For this review, take the finished solid that the model builds, in its own axes (mm). A direction names the side the tool comes from. Coordinates: 2 decimals unless noted, no trailing zeros. Write each loop counter-clockwise with the first axis right and the second up, starting at its lowest first coordinate (ties: lowest second). Pieces come first, ordered by that corner, then holes.
1) To check wall thickness, follow line 1 along Y through (x, z) = (69, 13); line 2 along Y through (x, z) = (42.5, 9); line 3 along Y through (x, z) = (98, 10). State the ranges of each line that lie inside material, in increasing order.
2) We need section A-A on x = 34.5. Write out the cut boundary in (y, z).
3) We need section C-C on y = -19. Write out the cut boundary in (x, z).
4) Mouldability with a two-part tool opening along Y and no side actions: class faces 4 (the face through (61.229, -27, -9)), 5 (the face through (19, -25.416, -7)), 6 (the face through (65, -20, -13.721)), 7 (the face through (65, 58.95, 14)) as pulls with the +Y half, pulls with the -Y half, needs draft (parallel to the pull), parting line crosses it, or undercut.
5) Insertion check: P1, Ø4, axis at x = 103, z = 23.5, coming from the +Y side; P2, Ø11.5, axis at x = 33.5, y = -24.5, coming from the +Z side; P3, Ø4, axis at x = 95, y = 44.5, coming from the +Z side. Each pin has a flat end and moves straight along its axis. Give the tip position at first contact, or say it passes through.
6) We need section B-B on z = 4.5. Write out the cut boundary in (x, y), then the cut area to 3 significant figures.
7) For faces 1 (the face through (113, -25.416, -7)), 2 (the face through (34, -22.914, -1)), 3 (the face through (59.601, -27, -9)), list the 3-axis set-ups (+Z, -Z, +X, -X, +Y, -Y) from which the entire face can be reached by the end or side of a thin tool; tool diameter is ignored.
8) We need section D-D on z = 30. Write out the cut boundary in (x, y).
from build123d import *

# Parameters (mm, degrees)
F1_DEPTH  = 132.11009
F2_W      = 132.11009
F2_H      = 1.6692737117
F3_DEPTH  = 14.2200058326
F4_W      = 5.6164497176
F4_H      = 5.6164497176
F5_DEPTH  = 24.97072611
F4_W_2    = 1.6288390616
F4_H_2    = 3.1137447804
F6_DEPTH  = 10
F7_W      = 3.1137447804
F7_H      = 1.2358725164
F8_DEPTH  = 57.6303704236
F9_W      = 3.1137447804
F9_H      = 1.2358725164
F10_DEPTH = 26.006960353


with BuildPart() as f1:
    # F0 (on Right) → F1 (new body)
    with BuildSketch(Plane.YZ):
        Polygon((-41.4899997413, 44.3699993193), (-28.5300053656, 44.3699993193), (58.9500032365, 44.3699993193), (71.9099976122, 44.3699993193), (15.2099989355, 73.1699988246), align=None)
        Polygon((-14.309999533, 11.2499995157), (-14.309999533, -15.3900003061), (58.9500032365, -15.3900003061), (58.9500032365, 44.3699993193), (-28.5300053656, 44.3699993193), (-28.5300053656, 11.2499995157), align=None)
    extrude(amount=F1_DEPTH)

    # F2 (on face) → F3 (join, through all)
    with BuildSketch(Plane.XZ.offset(14.309999533)):
        with Locations((66.055045, -14.5553634502)):
            Rectangle(F2_W, F2_H)
    extrude(amount=F3_DEPTH)

    # F4 (on face) → F5 (join, through all)
    with BuildSketch(Plane.XY.offset(-13.7207265943)):
        with Locations((2.8082248588, -25.7217805068)):
            Rectangle(F4_W, F4_H)
        with Locations((34.4316349294, -25.7217805068)):
            Rectangle(F4_W, F4_H)
        with Locations((66.055045, -25.7217805068)):
            Rectangle(F4_W, F4_H)
        with Locations((97.6784550706, -25.7217805068)):
            Rectangle(F4_W, F4_H)
        with Locations((129.3018651412, -25.7217805068)):
            Rectangle(F4_W, F4_H)
    extrude(amount=F5_DEPTH)

    # F4 (on face) → F6 (join)
    with BuildSketch(Plane.XY.offset(-13.7207265943)):
        with Locations((2.8082248588, -25.7217805068)):
            Rectangle(F4_W, F4_H)
        with Locations((34.4316349294, -25.7217805068)):
            Rectangle(F4_W, F4_H)
        with Locations((66.055045, -25.7217805068)):
            Rectangle(F4_W, F4_H)
        with Locations((97.6784550706, -25.7217805068)):
            Rectangle(F4_W, F4_H)
        with Locations((129.3018651412, -25.7217805068)):
            Rectangle(F4_W, F4_H)
        with Locations((8.4482542712, -26.9731329754)):
            Rectangle(F4_W_2, F4_H_2)
        with Locations((13.5340920827, -26.9731329754)):
            Rectangle(F4_W_2, F4_H_2)
        with Locations((18.6199298941, -26.9731329754)):
            Rectangle(F4_W_2, F4_H_2)
        with Locations((23.7057677055, -26.9731329754)):
            Rectangle(F4_W_2, F4_H_2)
        with Locations((28.791605517, -26.9731329754)):
            Rectangle(F4_W_2, F4_H_2)
        with Locations((45.1575021533, -26.9731329754)):
            Rectangle(F4_W_2, F4_H_2)
        with Locations((50.2433399647, -26.9731329754)):
            Rectangle(F4_W_2, F4_H_2)
        with Locations((55.3291777761, -26.9731329754)):
            Rectangle(F4_W_2, F4_H_2)
        with Locations((60.4150155876, -26.9731329754)):
            Rectangle(F4_W_2, F4_H_2)
        with Locations((40.0716643418, -26.9731329754)):
            Rectangle(F4_W_2, F4_H_2)
        with Locations((108.4043222945, -26.9731329754)):
            Rectangle(F4_W_2, F4_H_2)
        with Locations((113.4901601059, -26.9731329754)):
            Rectangle(F4_W_2, F4_H_2)
        with Locations((118.5759979173, -26.9731329754)):
            Rectangle(F4_W_2, F4_H_2)
        with Locations((123.6618357288, -26.9731329754)):
            Rectangle(F4_W_2, F4_H_2)
        with Locations((103.318484483, -26.9731329754)):
            Rectangle(F4_W_2, F4_H_2)
    extrude(amount=F6_DEPTH)

    # F7 (on face) → F8 (join, through all)
    with BuildSketch(Plane.YZ.offset(5.6164497176)):
        with Locations((-26.9731329754, -3.1027903361)):
            Rectangle(F7_W, F7_H)
    extrude(amount=F8_DEPTH)

    # F9 (on face) → F10 (join, through all)
    with BuildSketch(Plane.YZ.offset(100.4866799294)):
        with Locations((-26.9731329754, -3.1027903361)):
            Rectangle(F9_W, F9_H)
    extrude(amount=F10_DEPTH)


solid = f1.part
Result:
1. line 1: y = -28.53 to 58.95
1. line 2: y = -14.31 to 58.95
1. line 3: y = -28.53 to -22.91, -14.31 to 58.95
2. outline: (-41.49, 44.37) - (-28.53, 44.37) - (-28.53, -15.39) - (58.95, -15.39) - (58.95, 44.37) - (71.91, 44.37) - (15.21, 73.17) - close; hole (-22.91, -13.72) - (-14.31, -13.72) - (-14.31, 11.25) - (-22.91, 11.25) - close
3. outline: (0, -15.39) - (132.11, -15.39) - (132.11, -13.72) - (0, -13.72) - close; (0, 11.25) - (132.11, 11.25) - (132.11, 55.79) - (0, 55.79) - close
4. face 4: needs draft
4. face 5: undercut
4. face 6: undercut
4. face 7: pulls with the +Y half
5. P1: stops at y = 58.95
5. P2: stops at z = 55.92
5. P3: stops at z = 59.31
6. outline: (0, -28.53) - (5.62, -28.53) - (5.62, -22.91) - (0, -22.91) - close; (0, -14.31) - (132.11, -14.31) - (132.11, 58.95) - (0, 58.95) - close; (31.62, -28.53) - (37.24, -28.53) - (37.24, -22.91) - (31.62, -22.91) - close; (63.25, -28.53) - (68.86, -28.53) - (68.86, -22.91) - (63.25, -22.91) - close; (94.87, -28.53) - (100.49, -28.53) - (100.49, -22.91) - (94.87, -22.91) - close; (126.49, -28.53) - (132.11, -28.53) - (132.11, -22.91) - (126.49, -22.91) - close
6. area: 9,840 mm2
7. face 1: none
7. face 2: +X, -X
7. face 3: -Y
8. outline: (0, -28.53) - (132.11, -28.53) - (132.11, 58.95) - (0, 58.95) - close
